from build123d import *

# Parameters (mm, degrees)
SKETCH1_R           = 60
SKETCH1_R_2         = 4
SKETCH1_R_3         = 1.55
BOSS_EXTRUDE2_DEPTH = 8
SKETCH2_R           = 8
CUT_EXTRUDE1_DEPTH  = 5
SKETCH3_R           = 3.5
CUT_EXTRUDE2_DEPTH  = 3
SKETCH4_R           = 58
SKETCH4_R_2         = 56
BOSS_EXTRUDE3_DEPTH = 3


with BuildPart() as part:
    # Sketch1 → Boss-Extrude2 (new body)
    with BuildSketch(Plane.XY):
        Circle(SKETCH1_R)
        Circle(SKETCH1_R_2, mode=Mode.SUBTRACT)
        with Locations((-36.769552622, 36.769552622)):
            Circle(SKETCH1_R_3, mode=Mode.SUBTRACT)
        with Locations((0, 52)):
            Circle(SKETCH1_R_3, mode=Mode.SUBTRACT)
        with Locations((36.769552622, 36.769552622)):
            Circle(SKETCH1_R_3, mode=Mode.SUBTRACT)
        with Locations((52, 0)):
            Circle(SKETCH1_R_3, mode=Mode.SUBTRACT)
        with Locations((36.769552622, -36.769552622)):
            Circle(SKETCH1_R_3, mode=Mode.SUBTRACT)
        with Locations((0, -52)):
            Circle(SKETCH1_R_3, mode=Mode.SUBTRACT)
        with Locations((-36.769552622, -36.769552622)):
            Circle(SKETCH1_R_3, mode=Mode.SUBTRACT)
        with Locations((-52, 0)):
            Circle(SKETCH1_R_3, mode=Mode.SUBTRACT)
    extrude(amount=BOSS_EXTRUDE2_DEPTH)

    # Sketch2 → Cut-Extrude1 (cut)
    with BuildSketch(Plane.XY.offset(8)):
        Circle(SKETCH2_R)
    extrude(amount=-CUT_EXTRUDE1_DEPTH, mode=Mode.SUBTRACT)

    # Sketch3 → Cut-Extrude2 (cut)
    with BuildSketch(Plane.XY.offset(8)):
        with Locations((0, 52)):
            Circle(SKETCH3_R)
        with Locations((36.769552622, 36.769552622)):
            Circle(SKETCH3_R)
        with Locations((52, 0)):
            Circle(SKETCH3_R)
        with Locations((36.769552622, -36.769552622)):
            Circle(SKETCH3_R)
        with Locations((0, -52)):
            Circle(SKETCH3_R)
        with Locations((-36.769552622, -36.769552622)):
            Circle(SKETCH3_R)
        with Locations((-52, 0)):
            Circle(SKETCH3_R)
        with Locations((-36.769552622, 36.769552622)):
            Circle(SKETCH3_R)
    extrude(amount=-CUT_EXTRUDE2_DEPTH, mode=Mode.SUBTRACT)

    # Sketch4 → Boss-Extrude3 (add)
    with BuildSketch(Plane(origin=(0, 0, 0), x_dir=(-1, 0, 0), z_dir=(0, 0, -1))):
        with Locations(Location((0, 0, 0), (0, 0, 180))):
            Circle(SKETCH4_R)
        Circle(SKETCH4_R_2, mode=Mode.SUBTRACT)
    extrude(amount=BOSS_EXTRUDE3_DEPTH)


solid = part.part
Can you work these out from the model? Positions are in its coordinate system, mm. A direction names the side the tool comes from. Give positions to 0.01 mm unless a question says otherwise; leave off trailing zeros. Order: outer loops, then holes, each group sorted by start corner. A loop starts at its lowest first (then second) coordinate and runs counter-clockwise, first axis right, second up. Notation, with made-up numbers: M 59.5,64 L 88.5,64 A7 cw 88.5,74 Z; hole C -9,51.25 d6. An arc over 180 degrees is marked long. Use one line per item in the form item = value. Start each with the question number.
Item 1: If I drill on line 1 along Y through (x, z) = (0, 5.45); line 2 along X through (y, z) = (-2, 6.5); line 3 along Z through (x, y) = (-12, -9), over which ranges is the centre line in solid material (lowest first)?
Item 2: For faces 1 (the cylindrical face through (-0.867, -3.905, 1.479)), 2 (the flat face through (-36, -38.3, 5)), which set-ups out of +Z, -Z, +X, -X, +Y, -Y let a thin tool reach every point of the face, with its end or its side?
Item 3: If we section it at C-C (z = -1.5): Write out the boundary of the cut face in (x, y), then the cut area to 3 significant figures.
Item 4: If we section it at A-A (x = -52): Write out the boundary of the cut face in (y, z).
Item 5: Will these pins go through, and if not, where does the flat tip stop? pin 1 Ø1 at (y, z) = (11, 2.5) entering from +X; pin 2 Ø6 at (x, z) = (7.5, 6) entering from +Y; pin 3 Ø3.5 at (x, y) = (-52, 0) entering from +Z.
Item 6: We'd pull the mould along Y, two halves only. Please class faces 3 (the cylindrical face through (26.76, 51.46, -1.48)), 4 (the flat face through (12, 1, 8)), 5 (the cylindrical face through (36.434, 35.256, 2.465)): +Y half, -Y half, draft (parallel to the pull), parting line (faces both ways), or undercut.
Item 7: If we section it at B-B (y = 0): State how many separate pieces and enclosed holes the cut face has, then the cut area to 3 significant figures.
Outcome:
q1.line_1 = -60 to -55.5, -48.5 to -8, 8 to 48.5, 55.5 to 60
q1.line_2 = -59.97 to -54.87, -49.13 to -7.75, 7.75 to 49.13, 54.87 to 59.97
q1.line_3 = 0 to 8
q2.face_1 = +Z, -Z
q2.face_2 = +Z
q3.outline = C 0,0 d116; hole C 0,0 d112
q3.area = 716 mm2
q4.outline = M -29.93,0 L -25.69,0 L -25.69,-3 L -20.78,-3 L -20.78,0 L -1.55,0 L -1.55,5 L -3.5,5 L -3.5,8 L -29.93,8 Z; M 1.55,0 L 20.78,0 L 20.78,-3 L 25.69,-3 L 25.69,0 L 29.93,0 L 29.93,8 L 3.5,8 L 3.5,5 L 1.55,5 Z
q5.pin_1 = 59.07
q5.pin_2 = 59.83
q5.pin_3 = 5
q6.face_3 = parting line
q6.face_4 = draft
q6.face_5 = undercut
q7.separate_pieces = 4
q7.enclosed_holes = 0
q7.area = 795 mm2
